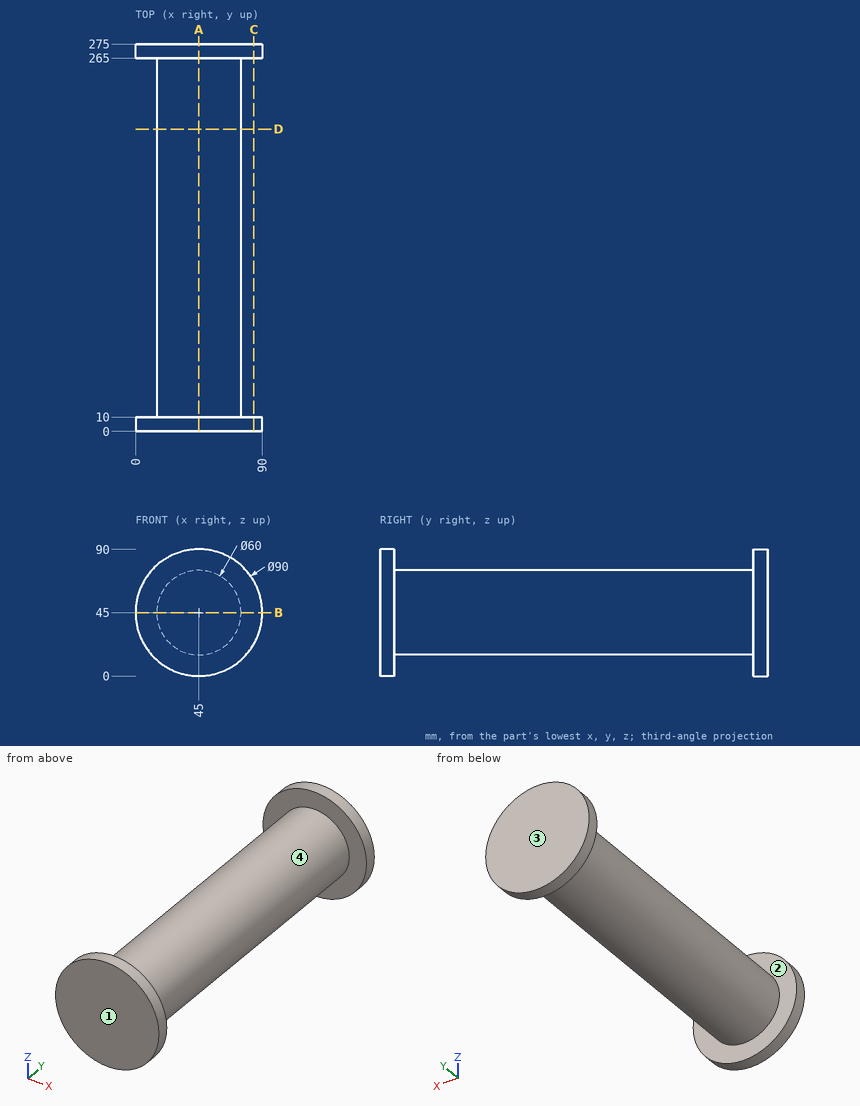
Input: dimensioned drawing with shaded views. Units: mm. Origin: part minimum x, y, z. Round coordinates to 2 decimals unless told otherwise and drop trailing zeros. Loops run counter-clockwise (first coordinate to the right, second up) from the corner with the lowest first, then second, coordinate; pieces in that order, holes last. Notation, with made-up numbers: (8, -19) -> (43, -19) arc R22 ccw to (43, -8) -> close; hole circle Ø10 at (79, -13). An arc over 180 degrees is marked (long way). Use one line per item in the form item = value. Start each with the question number.
1) First-contact query: P1, Ø3, axis at x = 29, y = 60.5, coming from the -Z side; P2, Ø4, axis at x = 70, y = 50, coming from the +Z side; P3, Ø4, axis at y = 137, z = 58.5, coming from the -X side. Flat tips, straight axial feed; report the tip coordinate or a pass-through.
2) Section B-B on z = 45. Output: boundary loops of the cut face in (x, y), then the cut area to 3 significant figures.
3) Line query: L1, parallel to Y at x = 49.5, z = 81.5; L2, parallel to Z at x = 17.5, y = 196; L3, parallel to Z at x = 71, y = 255.5. Output: solid intervals per line, ascending.
4) Section D-D on y = 214.5. Output: boundary loops of the cut face in (x, z).
5) Section C-C on x = 84. Output: boundary loops of the cut face in (y, z), then the cut area to 3 significant figures.
6) Draft query along Y for the marked faces 1, 2, 3 and 4. Return one class per face: released by +Y, released by -Y, zero draft, split by the parting line, or undercut.
7) Section A-A on x = 45. Output: boundary loops of the cut face in (y, z), then the cut area to 3 significant figures.
Response:
q1.P1 = 18.74
q1.P2 = 64.26
q1.P3 = 17.29
q2.outline = (0, 0) -> (90, 0) -> (90, 10) -> (75, 10) -> (75, 265) -> (90, 265) -> (90, 275) -> (0, 275) -> (0, 265) -> (15, 265) -> (15, 10) -> (0, 10) -> close
q2.area = 17,100 mm^2
q3.L1 = 0 to 10, 265 to 275
q3.L2 = 33.01 to 56.99
q3.L3 = 30.03 to 59.97
q4.outline = circle Ø60 at (45, 45)
q5.outline = (0, 22.55) -> (10, 22.55) -> (10, 67.45) -> (0, 67.45) -> close; (265, 22.55) -> (275, 22.55) -> (275, 67.45) -> (265, 67.45) -> close
q5.area = 898 mm^2
q6.face_1 = released by -Y
q6.face_2 = undercut
q6.face_3 = released by +Y
q6.face_4 = undercut
q7.outline = (0, 0) -> (10, 0) -> (10, 15) -> (265, 15) -> (265, 0) -> (275, 0) -> (275, 90) -> (265, 90) -> (265, 75) -> (10, 75) -> (10, 90) -> (0, 90) -> close
q7.area = 17,100 mm^2
